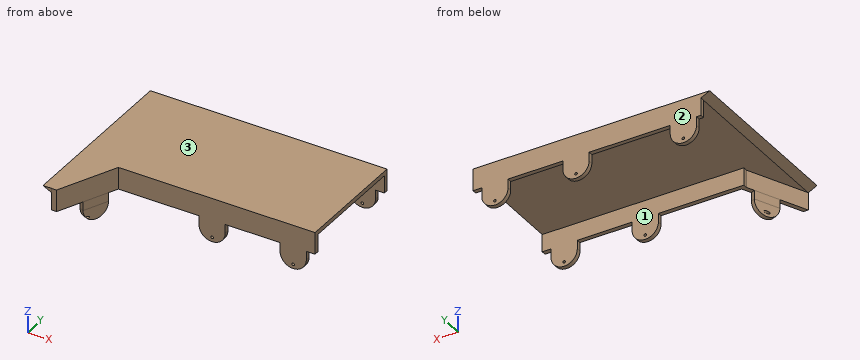
```python
from build123d import *

# Parameters (mm, degrees)
SKETCH1_W                                  = 260
SKETCH1_H                                  = 134
BOSS_EXTRUDE1_DEPTH                        = 5
SKETCH2_W                                  = 260
SKETCH2_H                                  = 5
BOSS_EXTRUDE2_DEPTH                        = 20
SKETCH4_W                                  = 230
SKETCH4_H                                  = 5
BOSS_EXTRUDE3_DEPTH                        = 20
BOSS_EXTRUDE4_DEPTH                        = 5
SKETCH7_R                                  = 1.5
CUT_EXTRUDE1_DEPTH                         = 5
BOSS_EXTRUDE5_DEPTH                        = 5
BOSS_EXTRUDE9_DEPTH                        = 25
BOSS_EXTRUDE10_DEPTH                       = 200
BOSS_EXTRUDE11_DEPTH                       = 5
SKETCH14_R                                 = 1.5
CUT_EXTRUDE2_DEPTH                         = 5
BOSS_EXTRUDE12_DEPTH                       = 10
BOSS_EXTRUDE13_DEPTH                       = 5
SKETCH19_R                                 = 1.5
CUT_EXTRUDE4_DEPTH                         = 307.022874962
CUT_EXTRUDE4_DEPTH_BACK                    = 307.022874962
MIRROR4_AT_THE_SECOND_PLANE_COPY_1_DEPTH   = 5
MIRROR4_AT_THE_SECOND_PLANE_COPY_2_SKETC_R = 1.5
MIRROR4_AT_THE_SECOND_PLANE_COPY_2_DEPTH   = 5


with BuildPart() as part:
    # Sketch1 → Boss-Extrude1 (new body)
    with BuildSketch(Plane.XY):
        with Locations((130, -67)):
            Rectangle(SKETCH1_W, SKETCH1_H)
    extrude(amount=BOSS_EXTRUDE1_DEPTH)

    # Sketch2 → Boss-Extrude2 (add)
    with BuildSketch(Plane(origin=(0, 0, 0), x_dir=(-1, 0, 0), z_dir=(0, 0, -1))):
        with Locations((-130, -2.5)):
            Rectangle(SKETCH2_W, SKETCH2_H)
    extrude(amount=BOSS_EXTRUDE2_DEPTH)

    # Sketch4 → Boss-Extrude3 (add)
    with BuildSketch(Plane(origin=(0, 0, 0), x_dir=(-1, 0, 0), z_dir=(0, 0, -1))):
        with Locations((-145, -131.5)):
            Rectangle(SKETCH4_W, SKETCH4_H)
    extrude(amount=BOSS_EXTRUDE3_DEPTH)

    # Sketch6 → Boss-Extrude4 (add)
    with BuildSketch(Plane(origin=(0, 0, 0), x_dir=(1, 0, 0), z_dir=(0, 1, 0))):
        with BuildLine():
            Line((5, 20), (5, 30))
            ThreePointArc((5, 30), (20, 45), (35, 30))
            Line((35, 30), (35, 20))
            Line((35, 20), (5, 20))
        make_face()
    extrude(amount=-BOSS_EXTRUDE4_DEPTH)

    # Sketch7 → Cut-Extrude1 (cut)
    with BuildSketch(Plane(origin=(0, 0, 0), x_dir=(1, 0, 0), z_dir=(0, 1, 0))):
        with Locations(Location((20, 40, 0), (0, 0, 270))):
            Circle(SKETCH7_R)
    extrude(amount=-CUT_EXTRUDE1_DEPTH, mode=Mode.SUBTRACT)

    # Sketch8 → Boss-Extrude5 (add)
    with BuildSketch(Plane(origin=(0, 0, 0), x_dir=(-1, 0, 0), z_dir=(0, 0, -1))):
        Polygon((-30, -134), (0, -200), (0, -134), align=None)
    extrude(amount=-BOSS_EXTRUDE5_DEPTH)

    # Sketch10 → Boss-Extrude9 (add)
    with BuildSketch(Plane.XY.offset(5)):
        Polygon((30, -134), (35.492293624, -134), (5.469823482, -200.049434314), (-0.022470143, -200.049434314), align=None)
    extrude(amount=-BOSS_EXTRUDE9_DEPTH)

    # Sketch11 → Boss-Extrude10 (add)
    with BuildSketch(Plane(origin=(0, 0, 0), x_dir=(1, 0, 0), z_dir=(0, 1, 0))):
        Polygon((0, 0), (-10, -5), (0, -5), align=None)
    extrude(amount=-BOSS_EXTRUDE10_DEPTH)

    # Sketch13 → Boss-Extrude11 (add)
    with BuildSketch(Plane(origin=(0, 0, 0), x_dir=(1, 0, 0), z_dir=(0, 1, 0))):
        with BuildLine():
            Line((220, 30), (220, 20))
            Line((220, 20), (250, 20))
            Line((250, 20), (250, 29.999997567))
            ThreePointArc((250, 29.999997567), (235.000001217, 44.999997567), (220, 30))
        make_face()
    boss_extrude11 = extrude(amount=-BOSS_EXTRUDE11_DEPTH)

    # Sketch14 → Cut-Extrude2 (cut)
    with BuildSketch(Plane(origin=(0, 0, 0), x_dir=(1, 0, 0), z_dir=(0, 1, 0))):
        with Locations(Location((235, 39.999997567, 0), (0, 0, 270))):
            Circle(SKETCH14_R)
    cut_extrude2 = extrude(amount=-CUT_EXTRUDE2_DEPTH, mode=Mode.SUBTRACT)

    # Sketch15 → Boss-Extrude12 (add)
    with BuildSketch(Plane(origin=(0, 0, -20), x_dir=(-1, 0, 0), z_dir=(0, 0, -1))):
        Polygon((-30.758876552, -144.41351756), (-26.207044165, -142.344502838), (-13.792955835, -169.655497162), (-18.344788223, -171.724511883), align=None)
    extrude(amount=BOSS_EXTRUDE12_DEPTH)

    # Sketch17 → Boss-Extrude13 (add)
    with BuildSketch(Plane(origin=(75.342465753, -34.246575342, 0), x_dir=(0, 0, 1), z_dir=(-0.9103664774626048, 0.41380294430118403, 0))):
        with BuildLine():
            Line((-30, -118.741111598), (-30, -148.741111598))
            ThreePointArc((-30, -148.741111598), (-45, -133.741111598), (-30, -118.741111598))
        make_face()
    extrude(amount=-BOSS_EXTRUDE13_DEPTH)

    # Sketch19 → Cut-Extrude4 (cut, two sides)
    with BuildSketch(Plane(origin=(0, -155, 0), x_dir=(1, 0, 0), z_dir=(0, 1, 0))) as cut_extrude4_sk:
        with Locations(Location((20, 40, 0), (0, 0, 270))):
            Circle(SKETCH19_R)
    extrude(amount=CUT_EXTRUDE4_DEPTH, mode=Mode.SUBTRACT)
    extrude(cut_extrude4_sk.sketch, amount=-CUT_EXTRUDE4_DEPTH_BACK, mode=Mode.SUBTRACT)

    # Mirror4: Boss-Extrude11, Cut-Extrude2 across plane
    add(boss_extrude11.mirror(Plane.ZX.offset(-67)))
    add(cut_extrude2.mirror(Plane.ZX.offset(-67)), mode=Mode.SUBTRACT)

    # Mirror4 at the second plane: Boss-Extrude11, Cut-Extrude2 across plane
    add(boss_extrude11.mirror(Plane.ZY.offset(-188.75)))
    add(cut_extrude2.mirror(Plane.ZY.offset(-188.75)), mode=Mode.SUBTRACT)

    # Mirror4 at the second plane copy 1 sketc → Mirror4 at the second plane copy 1 (add)
    with BuildSketch(Plane(origin=(377.5, -134, 0), x_dir=(-1, 0, 0), z_dir=(0, -1, 0))):
        with BuildLine():
            Line((220, 30), (220, 20))
            Line((220, 20), (250, 20))
            Line((250, 20), (250, 29.999997567))
            ThreePointArc((250, 29.999997567), (235.000001217, 44.999997567), (220, 30))
        make_face()
    extrude(amount=-MIRROR4_AT_THE_SECOND_PLANE_COPY_1_DEPTH)

    # Mirror4 at the second plane copy 2 sketc → Mirror4 at the second plane copy 2 (cut)
    with BuildSketch(Plane(origin=(377.5, -134, 0), x_dir=(-1, 0, 0), z_dir=(0, -1, 0))):
        with Locations(Location((235, 39.999997567, 0), (0, 0, 270))):
            Circle(MIRROR4_AT_THE_SECOND_PLANE_COPY_2_SKETC_R)
    extrude(amount=-MIRROR4_AT_THE_SECOND_PLANE_COPY_2_DEPTH, mode=Mode.SUBTRACT)


solid = part.part
```
Read the model definition and answer for the solid it produces. Units are mm, in the model's axes. Face numbers are marked on the shaded views. Coordinates: 2 decimals unless noted, no trailing zeros. Loops run counter-clockwise (first coordinate to the right, second up) from the corner with the lowest first, then second, coordinate; pieces in that order, holes last.
(1) The part is cut by section B-B (z = -33). Determine the outline of the cut face in (x, y), and give its area (3 significant figures).
Solution:
outline: (5.3, -5) - (34.7, -5) - (34.7, 0) - (5.3, 0) - close; (13.92, -169.38) - (18.47, -171.45) - (30.63, -144.69) - (26.08, -142.62) - close; (127.8, -134) - (157.2, -134) - (157.2, -129) - (127.8, -129) - close; (127.8, -5) - (157.2, -5) - (157.2, 0) - (127.8, 0) - close; (220.3, -134) - (249.7, -134) - (249.7, -129) - (220.3, -129) - close; (220.3, -5) - (249.7, -5) - (249.7, 0) - (220.3, 0) - close
area: 882 mm2
(2) The part is cut by section D-D (y = -109). Determine the outline of the cut face in (x, z), and give its area (4 significant figures).
Solution:
outline: (-10, 5) - (0, 0) - (260, 0) - (260, 5) - close
area: 1,325 mm2
(3) Flat-ended cylindrical pins translate along their axes: pin 1 Ø12 at (y, z) = (-178, -14) entering from +X; pin 2 Ø1.5 at (x, y) = (185, -3.5) entering from -Z; pin 3 Ø1.8 at (x, z) = (20, -40) entering from -Y; pin 4 Ø5.5 at (y, z) = (-1.5, -6.5) entering from -X. Find the tip coordinate at first contact, or state that the pin passes through.
Solution:
pin 1: stops at x = 18.22
pin 2: stops at z = -20
pin 3: passes through
pin 4: stops at x = 0
(4) Consider line 1 along Y through (x, z) = (185.5, -3); line 2 along Z through (x, y) = (235, -130.15); line 3 along X through (y, z) = (-2.8, -40). Determine where each line is inside the solid, lowest interval first.
Solution:
line 1: y = -134 to -129, -5 to 0
line 2: z = -45 to -41.5, -38.5 to 5
line 3: x = 8.82 to 18.5, 21.5 to 31.18, 131.32 to 141, 144 to 153.68, 223.82 to 233.5, 236.5 to 246.18
(5) The mould has two halves that part along Y. Classify the marked faces 1, 2 and 3: released by +Y, released by -Y, zero draft, split by the parting line, or undercut.
Solution:
face 1: undercut
face 2: released by +Y
face 3: zero draft
(6) The part is cut by section C-C (x = 174.5). Determine the outline of the cut face in (y, z), and give its area (3 significant figures).
Solution:
outline: (-134, -20) - (-129, -20) - (-129, 0) - (-5, 0) - (-5, -20) - (0, -20) - (0, 5) - (-134, 5) - close
area: 870 mm2
(7) The part is cut by section A-A (z = -5.5). Determine the outline of the cut face in (x, y).
Solution:
outline: (-0.02, -200.05) - (5.47, -200.05) - (35.49, -134) - (260, -134) - (260, -129) - (30, -129) - (30, -134) - close; (0, -5) - (260, -5) - (260, 0) - (0, 0) - close
